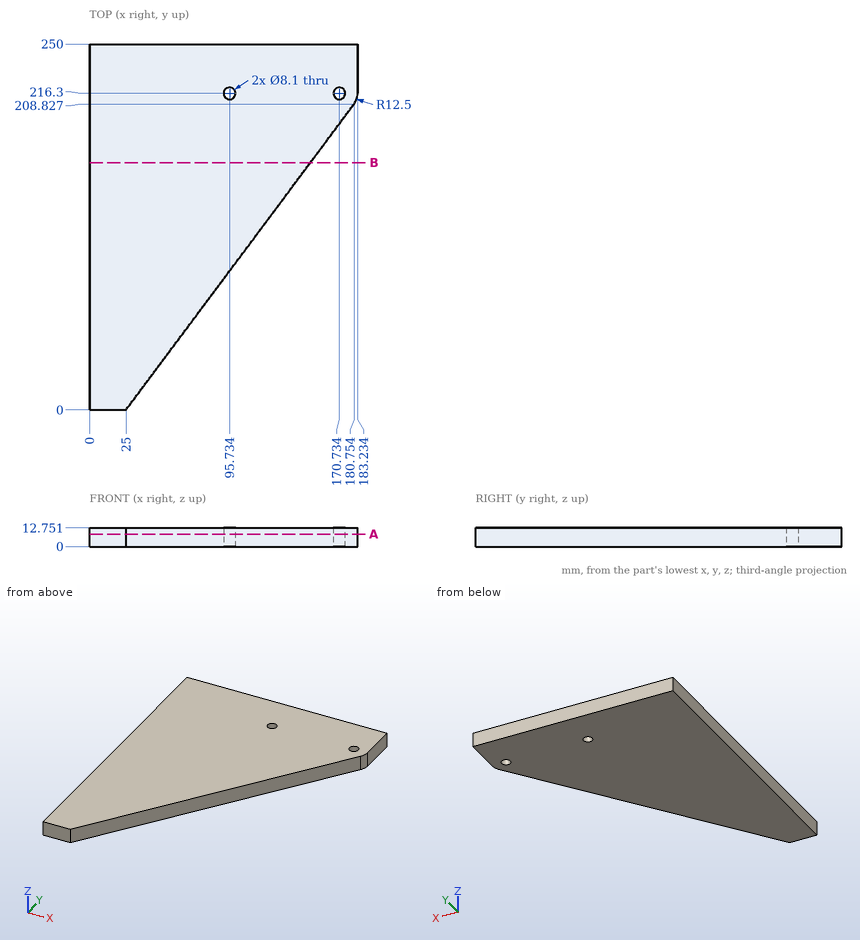
Answer from the drawing. Dimensions are ordinates in mm from the lowest x, y and z of the part. Give positions to 0.01 mm unless a question says otherwise; leave off trailing zeros. Loops run counter-clockwise (first coordinate to the right, second up) from the corner with the lowest first, then second, coordinate; pieces in that order, holes last.
Item 1: The part is cut by section A-A (z = 8.5). Write down the section's boundary in (x, y), and give its area (3 significant figures).
Item 2: This flat-tipped pin is pushed along its axis until it touches: pin 1 Ø13 at (x, y) = (95.734, 216.3) entering from -Z. Where does it stop, or does it pass through?
Item 3: The part is cut by section B-B (y = 169). Write down the section's boundary in (x, z), and give its area (3 significant figures).
Item 4: Find the intervals of material crossed by line 1 along X through (y, z) = (217, 8.25) (1 decimal); line 2 along Y through (x, z) = (167.5, 12) (1 decimal); line 3 along Y through (x, z) = (93.5, 2), in increasing order.
Taken from the geometry:
1. outline: (0, 0) - (25, 0) - (180.75, 208.83) arc R12.5 ccw to (183.23, 216.3) - (183.23, 250) - (0, 250) - close; hole circle Ø8.1 at (95.73, 216.3); hole circle Ø8.1 at (170.73, 216.3)
1. area: 28,900 mm2
2. pin 1: stops at z = 0
3. outline: (0, 0) - (151.05, 0) - (151.05, 12.75) - (0, 12.75) - close
3. area: 1,930 mm2
4. line 1: x = 0 to 91.7, 99.7 to 166.7, 174.7 to 183.2
4. line 2: y = 191.1 to 213.9, 218.7 to 250
4. line 3: y = 91.84 to 212.92, 219.68 to 250
